Read the model definition and answer for the solid it produces. Units are mm, in the model's axes. A direction names the side the tool comes from. Give positions to 0.01 mm unless a question says otherwise; leave off trailing zeros. Loops run counter-clockwise (first coordinate to the right, second up) from the corner with the lowest first, then second, coordinate; pieces in that order, holes last. Notation, with made-up numbers: (14, 45.5) - (63, 45.5) arc R26 ccw to (63, 69.5) - close; hole circle Ø2 at (-6, 13.5). An arc over 180 degrees is marked (long way). Put each result on its own line as item: value. Start each with the question number.
1. Given pin 1 Ø8.5 at (x, y) = (0.5, 1.5) entering from +Z; pin 2 Ø2.5 at (y, z) = (14, 4) entering from +X; pin 3 Ø4 at (y, z) = (12.5, 1) entering from +X; pin 4 Ø3 at (y, z) = (14.5, 5.5) entering from +X, each flat-ended and moving along its own axis, determine where each tip first touches the part or whether it passes through.
2. Consider L1, parallel to Z at x = -3, y = 14; L2, parallel to Z at x = -5, y = 15 (3 decimals); L3, parallel to Z at x = 1.25, y = 5. Determine where each line is inside the solid, lowest interval first. Write a range as from..to.
3. For a pull along Y with two mould halves and no side action, classify faces 4 (the cylindrical face through (-9.339, 12.476, 3.368)), 5 (the cylindrical face through (-1.85, -12.35, 4.07)), 6 (the flat face through (-8, -17.15, 4)), 7 (the flat face through (-8, -4, 8)) as released by +Y, released by -Y, zero draft, split by the parting line, or undercut.
4. A cutting plane is placed at B-B, the plane y = 14. Determine the outline of the cut face in (x, z) (3 decimals).
5. A cutting plane is placed at C-C, the plane z = 4.5. Count the separate pieces of the cut face and the enclosed holes in it, plus the area to 3 significant figures.
6. For faces 1 (the flat face through (-6, 15, 6.875)), 2 (the flat face through (-8, -3, 4)), 3 (the flat face through (5, 2, 1)), determine the directions among +Z, -Z, +X, -X, +Y, -Y from which every point of the face is accessible in a straight line to the end or side of a thin tool.
7. A cutting plane is placed at A-A, the plane x = -10. Determine the outline of the cut face in (y, z), plus the area to 3 significant figures.
```python
from build123d import *

# Parameters (mm, degrees)
F3_DEPTH = 8
F4_DEPTH = 1
F5_R     = 1.65
F6_DEPTH = 13.5965032877
F9_DEPTH = 2.8
F10_R    = 1.5
F11_R    = 3


# Not quite as in the source:
# - a pattern or mirror of a feature is missing from the dataset's text; its kind, count and spacing are read off the source's solid
# - a feature names something its author has since deleted; it is built from what else it names


with BuildPart() as f3:
    # F2 (on Top) → F3 (new body)
    with BuildSketch(Plane.XY):
        with BuildLine():
            Line((-11.41, 3), (-8.1131066799, 3))
            ThreePointArc((-8.1131066799, 3), (-0.999988831, 8.5920033949), (7.2072655829, 4.7830767104))
            Line((7.2072655829, 4.7830767104), (-1, 17.15))
            Line((-1, 17.15), (-11.41, 17.15))
            Line((-11.41, 17.15), (-11.41, 3))
        make_face()
        with BuildLine():
            ThreePointArc((7.2072655829, -4.7830767104), (-0.999988831, -8.5920033949), (-8.1131066799, -3))
            Line((-8.1131066799, -3), (-11.41, -3))
            Line((-11.41, -3), (-11.41, -17.15))
            Line((-11.41, -17.15), (-1, -17.15))
            Line((-1, -17.15), (7.2072655829, -4.7830767104))
        make_face()
        with BuildLine():
            ThreePointArc((-4.7877447718, 3), (1.5607277212, 5.430159204), (5.65, 0))
            ThreePointArc((5.65, 0), (1.5607277212, -5.430159204), (-4.7877447718, -3))
            Line((-4.7877447718, -3), (-8.1131066799, -3))
            ThreePointArc((-8.1131066799, -3), (-0.999988831, -8.5920033949), (7.2072655829, -4.7830767104))
            ThreePointArc((7.2072655829, -4.7830767104), (8.2814656702, -2.4979644421), (8.65, 0))
            ThreePointArc((8.65, 0), (8.2814656702, 2.4979644421), (7.2072655829, 4.7830767104))
            ThreePointArc((7.2072655829, 4.7830767104), (-0.999988831, 8.5920033949), (-8.1131066799, 3))
            Line((-8.1131066799, 3), (-4.7877447718, 3))
        make_face()
    extrude(amount=F3_DEPTH)

    # F2 (on Top) → F4 (join)
    with BuildSketch(Plane.XY):
        with BuildLine():
            ThreePointArc((-4.7877447718, -3), (1.5607277212, -5.430159204), (5.65, 0))
            ThreePointArc((5.65, 0), (1.5607277212, 5.430159204), (-4.7877447718, 3))
            Line((-4.7877447718, 3), (-3.9373214245, 3))
            ThreePointArc((-3.9373214245, 3), (1.5831549117, 4.6900021882), (4.95, 0))
            ThreePointArc((4.95, 0), (1.5831549117, -4.6900021882), (-3.9373214245, -3))
            Line((-3.9373214245, -3), (-4.7877447718, -3))
        make_face()
    extrude(amount=F4_DEPTH)

    # F5 (on face) → F6 (cut, through all)
    with BuildSketch(Plane(origin=(-11.41, 0, 0), x_dir=(0, -1, 0), z_dir=(-1, 0, 0))):
        with Locations((14, 4)):
            Circle(F5_R)
        with Locations((-14, 4)):
            Circle(F5_R)
    extrude(amount=-F6_DEPTH, mode=Mode.SUBTRACT)

    # F8 (on offset) → F9 (cut)
    with BuildSketch(Plane(origin=(-7.21, 0, 0), x_dir=(0, -1, 0), z_dir=(-1, 0, 0))):
        Polygon((17.15, 6.875), (15.6598820239, 6.875), (17.15, 4.2940399562), align=None)
        Polygon((17.15, 4.2940399562), (15.6598820239, 6.875), (12.3401179761, 6.875), (10.6802359522, 4), (12.3401179761, 1.125), (15.6598820239, 1.125), (17.15, 3.7059600438), align=None)
        Polygon((17.3197640478, 4), (17.15, 4.2940399562), (17.15, 3.7059600438), align=None)
        Polygon((17.15, 1.125), (17.15, 3.7059600438), (15.6598820239, 1.125), align=None)
    f9 = extrude(amount=-F9_DEPTH, mode=Mode.SUBTRACT)

    # F9_copies: F9 across plane
    add(f9.mirror(Plane.ZX), mode=Mode.SUBTRACT)

    # F10
    f10_edges = [f3.edges().sort_by_distance(p)[0] for p in [
        (5.65, 0, 8),
    ]]
    fillet(f10_edges, radius=F10_R)

    # F11
    f11_edges = [f3.edges().sort_by_distance(p)[0] for p in [
        (-1, -17.15, 4),
        (-1, 17.15, 4),
    ]]
    fillet(f11_edges, radius=F11_R)


solid = f3.part
```
Return value:
1. pin 1: stops at z = 7.21
1. pin 2: passes through
1. pin 3: stops at x = 3.41
1. pin 4: stops at x = 1.75
2. L1: z = 0..2.35, 5.65..8
2. L2: z = 0..1.125, 6.875..8
2. L3: z = 0..1
3. face 4: undercut
3. face 5: undercut
3. face 6: released by -Y
3. face 7: zero draft
4. outline: (-11.41, 0) - (1.09, 0) - (1.09, 2.35) - (-4.41, 2.35) - (-4.41, 1.125) - (-7.21, 1.125) - (-7.21, 2.35) - (-11.41, 2.35) - close; (-11.41, 5.65) - (-7.21, 5.65) - (-7.21, 6.875) - (-4.41, 6.875) - (-4.41, 5.65) - (1.09, 5.65) - (1.09, 8) - (-11.41, 8) - close
5. separate pieces: 5
5. enclosed holes: 0
5. area: 314 mm2
6. face 1: +Y
6. face 2: +Z, -Z, -X
6. face 3: +Z
7. outline: (-17.15, 0) - (-3, 0) - (-3, 8) - (-17.15, 8) - close; (3, 0) - (17.15, 0) - (17.15, 8) - (3, 8) - close; hole circle Ø3.3 at (-14, 4); hole circle Ø3.3 at (14, 4)
7. area: 209 mm2
